Source: CAD feature listing. Evaluate the final solid. Frame: model axes, mm. A direction names the side the tool comes from. Coordinates: 2 decimals unless noted, no trailing zeros. Order: outer loops, then holes, each group sorted by start corner. A loop starts at its lowest first (then second) coordinate and runs counter-clockwise, first axis right, second up. Notation, with made-up numbers: (12.5, 58) -> (52.5, 58) arc R27 cw to (52.5, 74) -> close; hole circle Ø7 at (9, -1). An arc over 180 degrees is marked (long way). Write item = value, one per line. Start each with the question number.
Item 1: Section query B-B (z = 1.7). Output: boundary loops of the cut face in (x, y).
Item 2: Ray query, line 1 along X through (y, z) = (-12.5, -0.35); line 2 along X through (y, z) = (-12.5, -0.9); line 3 along Z through (x, y) = (-10.5, -14). Return the intervals inside material, ascending. Write a range as [from, to].
Item 3: Section query A-A (y = -22.5). Output: boundary loops of the cut face in (x, z), then the cut area to 3 significant figures.
Item 4: Contact query for flat-ended pins moving along their axis: pin 1 (1.5 mm diameter, centred on y = -5.5, z = 0.5, fed in from -X); pin 2 (1 mm diameter, centred on y = -16.5, z = 1, fed in from -X); pin 3 (11 mm diameter, centred on x = 0, y = -12.5, fed in from -Z). Output: stop coordinate, or through.
Item 5: Set-up query: faces 1 (the conical face through (0.2, -12.8, -0.8)), 2 (the flat face through (0, -13, 2.4)). Return all of +Z, -Z, +X, -X, +Y, -Y with unobstructed straight access to the full face (end or side cutting, diameter ignored); none if empty.
Item 6: Mould query, pull axis X, two halves, no side actions, for faces 3 (the flat face through (-1, -22, 0)), 4 (the flat face through (12, -17, -0.6)), 5 (the conical face through (0, -21, -2)). Classes: released by +X, released by -X, zero draft, split by the parting line, or undercut.
Autodesk Inventor part; units mm, degrees
ref_plane "YZ Plane" through (0, 0, 0) normal (1, 0, 0) x (0, 1, 0)
ref_plane "XZ Plane" through (0, 0, 0) normal (0, 1, 0) x (-1, 0, 0)
ref_plane "XY Plane" through (0, 0, 0) normal (0, 0, 1) x (1, 0, 0)
sketch "Skizze1" plane through (0, 0, 0) normal (1, 0, 0) x (0, 1, 0)
  line L0 (0, 0) -> (0, -0.6)
  line L1 (-25, 0) -> (0, 0)
  line L2 (-25, -0.6) -> (0, -0.6)
  line L3 (-20.8023, -2.2) -> (-4.1977, -2.2)
  line L4 (-20.6011, -1.9989) -> (-21.4, -1.2)
  line L5 (-21.4, -1.2) -> (-21.4, 0)
  line L6 (-25, 0) -> (-25, -0.6)
  line L7 (-22.8485, -0.6) -> (-20.8497, -2.5989)
  line L8 (-21.0508, -2.8) -> (-3.9492, -2.8)
  line L9 (0, -0.6) -> (5, -0.6)
  line L10 (5, -0.6) -> (5, 2.4)
  line L11 (-12.5, -6.6891) -> (-12.5, -2.8)
  line L12 (0, 4.2178) -> (0, -8.5069)
  line L13 (5, 2.4) -> (-12.5, 2.4)
  line L14 (-19.2569, -1) -> (-5.7431, -1)
  line L15 (-18.5, -0.8) -> (-6.5, -0.8) construction
  line L16 (-6.5, -0.8) -> (-6.5, -1) construction
  line L17 (-6.5, -1) -> (-18.5, -1) construction
  line L18 (-18.5, -1) -> (-18.5, -0.8) construction
  line L19 (-18.5, -0.8) -> (-12.5, -0.9) construction
  line L20 (-6.5, -0.8) -> (-18.5, -1) construction
  line L21 (-12.5, 2.4) -> (-12.5, -0.8)
  line L22 (-12.5, -0.8) -> (-6.4, -0.7983) construction
  line L23 (-6.4, -0.7983) -> (-6.4, -1) construction
  line L24 (-12.5, -0.8) -> (-6.4, -0.7983) construction
  line L25 (-6.4, -0.7983) -> (-6.4, -1) construction
  line L26 (-12.5, -0.8) -> (-6.4, -0.7983)
  line L27 (-6.4, -0.7983) -> (-6.4, -1)
  line L28 (-6.5, -1) -> (-6.5167, -1)
  line L29 (-5.7431, -1) -> (-6.1949, -1.0051)
  line L30 (-3.6, 0) -> (0, 0)
  line L31 (-5.9715, -1.2285) -> (-6.1949, -1.0051)
  line L32 (-5, -2.2) -> (-4.4683, -2.2)
  line L33 (-5, -2.2) -> (-5.3167, -2.2)
  line L34 (-5.3167, -2.2) -> (-3.6196, -2.2) construction
  line L35 (-3.2, -1.2) -> (-3.2, 0)
  line L36 (-4.1989, -2.1989) -> (-3.2, -1.2)
  line L37 (-20.8023, -2.2) -> (-4.1977, -2.2)
  line L38 (-4.1977, -2.2) -> (-4.9977, -2.2)
  line L39 (-5.7431, -1) -> (-4.5431, -2.2)
  point P0 (-2.1515, -0.6)
  point P1 (-22.8485, -0.6)
  point P2 (-12.5, -1)
  point P3 (-12.5, -0.6)
  point P4 (-21.4, -0.6)
  point P5 (-12.5, 0)
  dimension "d0" = 5
  dimension "d1" = 3
  dimension "d2" = 17.1016
  dimension "d3" = 8.5508
  dimension "d4" = 12
  dimension "d5" = 0.2
  dimension "d6" = 6.1
revolve "Umdrehung1" add sketch "Skizze1" angle 360 about axis through (0, -12.5, 2.4) along (0, 0, -1) contours L12 L13 L10 L9 L0 | L1 L21 L13 L12 | L35 L2 L21 L1 | L35 L36 L3 L39 L14 L27 L26 L21 L2
equation "\"d3\" = 0.5 * d2"
properties part number "50_ETL_Membrane_Mould_Lower_v0"
Computed:
q1.outline = circle Ø35 at (0, -12.5)
q2.line_1 = [-17.5, -12.5], [-9.3, 9.3], [12.5, 17.5]
q2.line_2 = [-9.3, -6.1], [6.1, 9.3]
q2.line_3 = [0, 2.4]
q3.outline = (-14.36, -0.6) -> (-7.5, -0.6) -> (-7.5, 0) -> (7.5, 0) -> (7.5, -0.6) -> (14.36, -0.6) -> (14.36, 2.4) -> (-14.36, 2.4) -> close
q3.area = 77.2 mm^2
q4.pin_1 = -16.35
q4.pin_2 = -17.15
q4.pin_3 = -0.8
q5.face_1 = -Z
q5.face_2 = +Z, +X, -X, +Y, -Y
q6.face_3 = undercut
q6.face_4 = zero draft
q6.face_5 = split by the parting line
